The model under review builds one solid part; all positions refer to its coordinate system, in mm. Face numbers are marked on the shaded views. A direction names the side the tool comes from. Give positions to 0.01 mm unless a question says otherwise; leave off trailing zeros. Write each loop counter-clockwise with the first axis right and the second up, starting at its lowest first coordinate (ties: lowest second). Pieces come first, ordered by that corner, then holes.
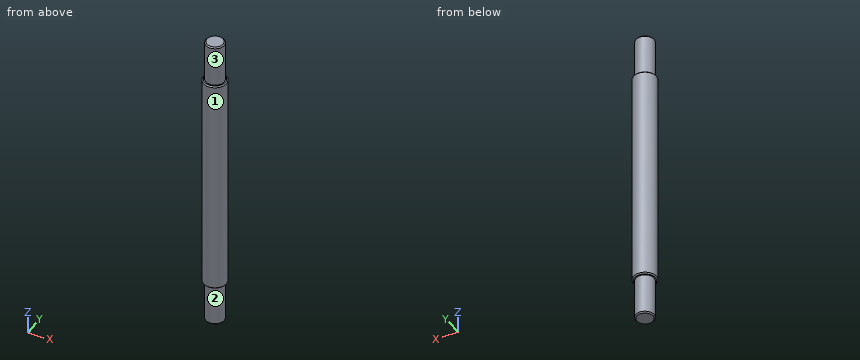
Autodesk Inventor part; units mm, degrees
ref_plane "YZ Plane" through (0, 0, 0) normal (1, 0, 0) x (0, 1, 0)
ref_plane "XZ Plane" through (0, 0, 0) normal (0, 1, 0) x (-1, 0, 0)
ref_plane "XY Plane" through (0, 0, 0) normal (0, 0, 1) x (1, 0, 0)
sketch "Sketch1" plane through (0, 0, 0) normal (0, 1, 0) x (-1, 0, 0)
  line L0 (1, 0) -> (-6, 0)
  line L1 (0, -93.1) -> (0, 93.1)
  line L2 (0, -66.5) -> (-4, -66.5)
  line L3 (-4, -66.5) -> (-4, -48.5)
  line L4 (-4, -48.5) -> (-5, -48.5)
  line L5 (-5, -48.5) -> (-5, 48.5)
  line L6 (-5, 48.5) -> (-4, 48.5)
  line L7 (-4, 48.5) -> (-4, 66.5)
  line L8 (-4, 66.5) -> (0, 66.5)
  dimension "d1" = 18
  dimension "d2" = 8
  dimension "d3" = 10
  dimension "d5" = 8
  dimension "d8" = 18
  dimension "d9" = 97
revolve "Revolution1" add sketch "Sketch1" angle 360 about axis through (0, 0, -10) along (0, 0, 1)
chamfer "Chamfer1" distance 0.5 angle 45 4 edges at (-4, 0, -66.5) (-4, 0, 66.5) (-5, 0, 48.5) (-5, 0, -48.5)
thread "Thread1"
thread "Thread2"
equation "\"d5\" = d2"
equation "\"d8\" = d1"
properties part number "Rear Wheel Axle"
1) Consider section C-C, the plane z = 38. Give the boundary of the cut face in (x, y), then the cut area to 3 significant figures.
2) Tool access review of the marked faces 1, 2 and 3: name each direction out of +Z, -Z, +X, -X, +Y, -Y from which nothing blocks a thin tool from reaching the whole face with its end or side.
3) Insertion check: pin 1 (1 mm diameter, centred on x = -3, y = -3.5, fed in from +Z). The pin has a flat end and moves straight along its axis. Give the tip position at first contact, or say it passes through.
4) To check wall thickness, follow probe 1 along Y at (x, z) = (-0.25, -50); probe 2 along X at (y, z) = (0.5, 21); probe 3 along Z at (x, y) = (0.5, 4). State the ranges of each line that lie inside material, in increasing order.
5) Consider section A-A, the plane x = 0. Give the boundary of the cut face in (y, z), then the cut area to 3 significant figures.
Answer block:
1. outline: circle Ø10 at (0, 0)
1. area: 78.5 mm2
2. face 1: +Z, -Z
2. face 2: -Z
2. face 3: +Z
3. pin 1: stops at z = 48.5
4. probe 1: y = -3.99 to 3.99
4. probe 2: x = -4.97 to 4.97
4. probe 3: z = -48.5 to 48.5
5. outline: (-5, -48) - (-4.5, -48.5) - (-4, -48.5) - (-4, -66) - (-3.5, -66.5) - (3.5, -66.5) - (4, -66) - (4, -48.5) - (4.5, -48.5) - (5, -48) - (5, 48) - (4.5, 48.5) - (4, 48.5) - (4, 66) - (3.5, 66.5) - (-3.5, 66.5) - (-4, 66) - (-4, 48.5) - (-4.5, 48.5) - (-5, 48) - close
5. area: 1,260 mm2
